from build123d import *

# Parameters (mm, degrees)
CROQUIS1_W              = 70.164619522
CROQUIS1_H              = 70.068399122
CROQUIS1_R              = 35
CROQUIS1_R_2            = 29
SALIENTE_EXTRUIR1_DEPTH = 3
REDONDEO1_R             = 10
CROQUIS2_R              = 3
CORTAR_EXTRUIR1_DEPTH   = 10


with BuildPart() as part:
    # Croquis1 → Saliente-Extruir1 (new body)
    # profile 1 of 2: a face of its own
    with BuildSketch(Plane.XY):
        Rectangle(CROQUIS1_W, CROQUIS1_H)
        Circle(CROQUIS1_R, mode=Mode.SUBTRACT)
    # profile 2 of 2: a face of its own
    with BuildSketch(Plane.XY):
        Circle(CROQUIS1_R)
        Circle(CROQUIS1_R_2, mode=Mode.SUBTRACT)
    extrude(amount=SALIENTE_EXTRUIR1_DEPTH)

    # Redondeo1
    redondeo1_edges = [part.edges().sort_by_distance(p)[0] for p in [
        (35.082309761, -35.034199561, 1.5),
        (-35.082309761, -35.034199561, 1.5),
        (-35.082309761, 35.034199561, 1.5),
        (35.082309761, 35.034199561, 1.5),
    ]]
    fillet(redondeo1_edges, radius=REDONDEO1_R)

    # Croquis2 → Cortar-Extruir1 (cut)
    with BuildSketch(Plane(origin=(0, 0, 0), x_dir=(-1, 0, 0), z_dir=(0, 0, -1))):
        with Locations((-27.082309761, 27.034199561)):
            Circle(CROQUIS2_R)
        with Locations((27.082309761, 27.034199561)):
            Circle(CROQUIS2_R)
        with Locations((-27.082309761, -27.034199561)):
            Circle(CROQUIS2_R)
        with Locations((27.082309761, -27.034199561)):
            Circle(CROQUIS2_R)
    extrude(amount=-CORTAR_EXTRUIR1_DEPTH, mode=Mode.SUBTRACT)


solid = part.part
Work out the finished part from the listing and answer in its coordinate system (mm). Give positions to 0.01 mm unless a question says otherwise; leave off trailing zeros. Loops run counter-clockwise (first coordinate to the right, second up) from the corner with the lowest first, then second, coordinate; pieces in that order, holes last. Notation, with made-up numbers: (-14, -36.5) - (37, -36.5) arc R25 cw to (37, 1.5) - close; hole circle Ø4 at (-22, 67.25). An arc over 180 degrees is marked (long way). Answer in a Markdown table with one row per item. Add a question column.
Q1. Determine the mould class of faces 1 (the cylindrical face through (32.08, -32.18, 1.52)), 2 (the cylindrical face through (-28.695, -24.505, 1.479)), 3 (the cylindrical face through (-32.23, -32.03, 1.52)) for opening direction X: released by +X, released by -X, zero draft, split by the parting line, or undercut.
Q2. The part is cut by section B-B (x = 0). Determine the outline of the cut face in (y, z), and give its area (3 significant figures).
Q3. The part is cut by section A-A (y = 0). Determine the outline of the cut face in (x, z).
Q4. Consider line 1 along X through (y, z) = (25, 2.5); line 2 along X through (y, z) = (1, 2.9); line 3 along Y through (x, z) = (26.5, 2.75). Determine where each line is inside the solid, lowest interval first.
Q5. The part is cut by section C-C (z = 1.6). Determine the outline of the cut face in (x, y).
Q6. This flat-tipped pin is pushed along its axis until it touches: P1, Ø1, axis at x = 27.5, y = 6.5, coming from the -Z side. Where does it stop, or does it pass through?
Solution:
| question | item | result |
|---|---|---|
| 1 | face 1 | released by +X |
| 1 | face 2 | undercut |
| 1 | face 3 | released by -X |
| 2 | outline | (-35.03, 0) - (-29, 0) - (-29, 3) - (-35.03, 3) - close; (29, 0) - (35.03, 0) - (35.03, 3) - (29, 3) - close |
| 2 | area | 36.2 mm² |
| 3 | outline | (-35.08, 0) - (-29, 0) - (-29, 3) - (-35.08, 3) - close; (29, 0) - (35.08, 0) - (35.08, 3) - (29, 3) - close |
| 4 | line 1 | x = -35.08 to -29.29, -24.88 to -14.7, 14.7 to 24.88, 29.29 to 35.08 |
| 4 | line 2 | x = -35.08 to -28.98, 28.98 to 35.08 |
| 4 | line 3 | y = -34.93 to -29.98, -24.09 to -11.78, 11.78 to 24.09, 29.98 to 34.93 |
| 5 | outline | (-35.08, -25.03) arc R10 ccw to (-25.08, -35.03) - (25.08, -35.03) arc R10 ccw to (35.08, -25.03) - (35.08, 25.03) arc R10 ccw to (25.08, 35.03) - (-25.08, 35.03) arc R10 ccw to (-35.08, 25.03) - close; hole circle Ø6 at (-27.08, -27.03); hole circle Ø6 at (-27.08, 27.03); hole circle Ø58 at (0, 0); hole circle Ø6 at (27.08, -27.03); hole circle Ø6 at (27.08, 27.03) |
| 6 | P1 | passes through |
